Geometry check sheet. Reference: the model listing, model coordinates, mm. Face numbers are marked on the shaded views. A direction names the side the tool comes from. Coordinates: 2 decimals unless noted, no trailing zeros. Order: outer loops, then holes, each group sorted by start corner. A loop starts at its lowest first (then second) coordinate and runs counter-clockwise, first axis right, second up. Notation, with made-up numbers: M -28,44 L -20,44 A27 cw -20,82 Z; hole C 21.25,-1 d4. An arc over 180 degrees is marked long. One line per item, written item: value. Start each with the question number.
1) Thickness scan on L1, parallel to Y at x = 0, z = 14; L2, parallel to X at y = 22, z = 7; L3, parallel to Y at x = 0, z = 58. Record the ranges inside material, lowest first. Write a range as from..to.
2) Access from +Z, -Z, +X, -X, +Y, -Y to the whole of each face (thin tool, end or side, straight path). Record for the marked faces 4 and 5.
3) Go/stop test with flat-tipped pins: P1, Ø4, axis at x = 23, z = 36, coming from the +Y side; P2, Ø14.5, axis at x = 0, y = 0, coming from the -Z side; P3, Ø6.5, axis at x = -10, y = -22, coming from the +Z side; P4, Ø2.5, axis at x = 10, y = -22, coming from the -Z side. Record where each tip stops, or that it passes through.
4) Sectioned sample at A-A, the plane y = 0. Enter the section's corners in (x, z), then the cut area to 3 significant figures.
5) Sectioned sample at D-D, the plane z = 61. Enter the section's corners in (x, y), then the cut area to 3 significant figures.
6) Sectioned sample at B-B, the plane x = -1. Enter the section's corners in (y, z), then the cut area to 3 significant figures.
7) Draft check along X on the marked faces 1, 2 and 3. Enter one of: pulls with the +X half, pulls with the -X half, needs draft (parallel to the pull), parting line crosses it, or undercut.
8) Sectioned sample at C-C, the plane z = 23. Enter the section's corners in (x, y).
```python
from build123d import *

# Parameters (mm, degrees)
SKETCH5_R                 = 34
BOSS_EXTRUDE1_DEPTH       = 70
SKETCH6_R                 = 27.5
CUT_EXTRUDE1_DEPTH        = 40
SKETCH7_R                 = 21.5
CUT_EXTRUDE2_DEPTH        = 10
SKETCH8_R                 = 12
CUT_EXTRUDE3_DEPTH        = 20
SKETCH9_R                 = 1.5
CUT_EXTRUDE4_DEPTH        = 20
M5X0_8_TAPPED_HOLE1_D     = 4.2
M5X0_8_TAPPED_HOLE1_DEPTH = 10
M5X0_8_TAPPED_HOLE1_TIP   = 1.2618073


with BuildPart() as part:
    # Sketch5 → Boss-Extrude1 (new body)
    with BuildSketch(Plane.XY):
        Circle(SKETCH5_R)
    extrude(amount=BOSS_EXTRUDE1_DEPTH)

    # Sketch6 → Cut-Extrude1 (cut)
    with BuildSketch(Plane.XY.offset(70)):
        Circle(SKETCH6_R)
    extrude(amount=-CUT_EXTRUDE1_DEPTH, mode=Mode.SUBTRACT)

    # Sketch7 → Cut-Extrude2 (cut)
    with BuildSketch(Plane.XY.offset(30)):
        Circle(SKETCH7_R)
    extrude(amount=-CUT_EXTRUDE2_DEPTH, mode=Mode.SUBTRACT)

    # Sketch8 → Cut-Extrude3 (cut)
    with BuildSketch(Plane(origin=(0, 0, 0), x_dir=(-1, 0, 0), z_dir=(0, 0, -1))):
        Circle(SKETCH8_R)
    extrude(amount=-CUT_EXTRUDE3_DEPTH, mode=Mode.SUBTRACT)

    # Sketch9 → Cut-Extrude4 (cut)
    with BuildSketch(Plane.XY.offset(70)):
        with Locations((-30.75, 0)):
            Circle(SKETCH9_R)
        with Locations((30.75, 0)):
            Circle(SKETCH9_R)
    extrude(amount=-CUT_EXTRUDE4_DEPTH, mode=Mode.SUBTRACT)

    # M5x0.8 Tapped Hole1
    with Locations(Plane(origin=(0, 0, 0), x_dir=(-1, 0, 0), z_dir=(0, 0, -1))):
        with Locations((-10, 22), (10, 22), (10, -22), (-10, -22)):
            Hole(M5X0_8_TAPPED_HOLE1_D / 2, depth=M5X0_8_TAPPED_HOLE1_DEPTH)
            with Locations((0, 0, -(M5X0_8_TAPPED_HOLE1_DEPTH + M5X0_8_TAPPED_HOLE1_TIP / 2))):  # 118° drill point
                Cone(0, M5X0_8_TAPPED_HOLE1_D / 2, M5X0_8_TAPPED_HOLE1_TIP, mode=Mode.SUBTRACT)


solid = part.part
```
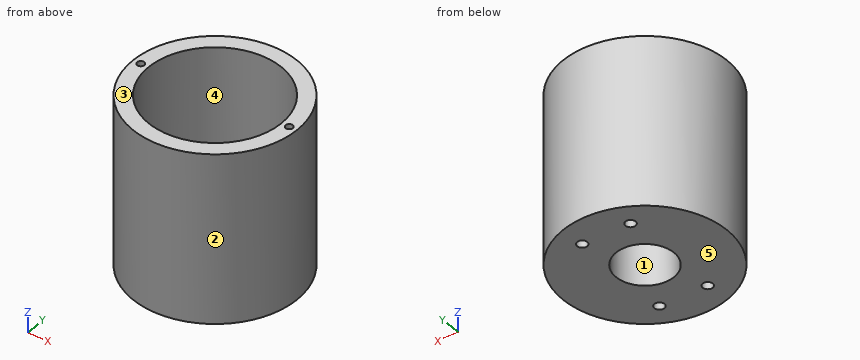
Final values:
1. L1: y = -34..-12, 12..34
1. L2: x = -25.92..-12.1, -7.9..7.9, 12.1..25.92
1. L3: y = -34..-27.5, 27.5..34
2. face 4: +Z
2. face 5: -Z, +X, -X, +Y, -Y
3. P1: stops at y = 26.74
3. P2: passes through
3. P3: stops at z = 30
3. P4: stops at z = 10.51
4. outline: M -34,0 L -12,0 L -12,20 L -21.5,20 L -21.5,30 L -27.5,30 L -27.5,70 L -29.25,70 L -29.25,50 L -32.25,50 L -32.25,70 L -34,70 Z; M 12,0 L 34,0 L 34,70 L 32.25,70 L 32.25,50 L 29.25,50 L 29.25,70 L 27.5,70 L 27.5,30 L 21.5,30 L 21.5,20 L 12,20 Z
4. area: 1,530 mm^2
5. outline: C 0,0 d68; hole C -30.75,0 d3; hole C 0,0 d55; hole C 30.75,0 d3
5. area: 1,240 mm^2
6. outline: M -33.99,0 L -11.96,0 L -11.96,20 L -21.48,20 L -21.48,30 L -27.48,30 L -27.48,70 L -33.99,70 Z; M 11.96,0 L 33.99,0 L 33.99,70 L 27.48,70 L 27.48,30 L 21.48,30 L 21.48,20 L 11.96,20 Z
6. area: 1,650 mm^2
7. face 1: undercut
7. face 2: parting line crosses it
7. face 3: needs draft
8. outline: C 0,0 d68; hole C 0,0 d43
